from build123d import *

# Parameters (mm, degrees)
ESQUISSE1_W                = 67
ESQUISSE1_H                = 18
BOSS_EXTRU_1_DEPTH         = 3
ESQUISSE2_W                = 10
ESQUISSE2_H                = 3
ENL_V_MAT_EXTRU_1_DEPTH    = 10
R_P_TITION_LIN_AIRE1_COUNT = 4
R_P_TITION_LIN_AIRE1_PITCH = 20
ESQUISSE3_W                = 3
ESQUISSE3_H                = 10
ENL_V_MAT_EXTRU_2_DEPTH    = 10
ESQUISSE4_W                = 3
ESQUISSE4_H                = 10
BOSS_EXTRU_2_DEPTH         = 3


with BuildPart() as part:
    # Esquisse1 → Boss.-Extru.1 (new body)
    with BuildSketch(Plane.XY):
        with Locations((33.5, -9)):
            Rectangle(ESQUISSE1_W, ESQUISSE1_H)
    extrude(amount=BOSS_EXTRU_1_DEPTH)

    # Esquisse2 → Enlèv. mat.-Extru.1 (cut)
    with BuildSketch(Plane.XY.offset(3)):
        with Locations((5, -16.5)):
            Rectangle(ESQUISSE2_W, ESQUISSE2_H)
    enl_v_mat_extru_1 = extrude(amount=-ENL_V_MAT_EXTRU_1_DEPTH, mode=Mode.SUBTRACT)

    # Répétition linéaire1: Enlèv. mat.-Extru.1 ×4
    with Locations(*[(i * R_P_TITION_LIN_AIRE1_PITCH, 0, 0) for i in range(1, R_P_TITION_LIN_AIRE1_COUNT)]):
        add(enl_v_mat_extru_1, mode=Mode.SUBTRACT)

    # Esquisse3 → Enlèv. mat.-Extru.2 (cut)
    with BuildSketch(Plane.XY.offset(3)):
        with Locations((65.5, -5)):
            Rectangle(ESQUISSE3_W, ESQUISSE3_H)
    extrude(amount=-ENL_V_MAT_EXTRU_2_DEPTH, mode=Mode.SUBTRACT)

    # Esquisse4 → Boss.-Extru.2 (add)
    with BuildSketch(Plane.ZY):
        with Locations((1.5, -5)):
            Rectangle(ESQUISSE4_W, ESQUISSE4_H)
    extrude(amount=BOSS_EXTRU_2_DEPTH)


solid = part.part
The listing builds one solid part. Answer for the finished solid, in the listing's coordinates (mm). A direction names the side the tool comes from. Give positions to 0.01 mm unless a question says otherwise; leave off trailing zeros. Write each loop counter-clockwise with the first axis right and the second up, starting at its lowest first coordinate (ties: lowest second). Pieces come first, ordered by that corner, then holes. Notation, with made-up numbers: (62, -40) -> (97, -40) arc R31 ccw to (97, -4) -> close; hole circle Ø1 at (56.5, 33.5). An arc over 180 degrees is marked (long way). Use a Markdown table: item, result.
(1) For faces 4 (the flat face through (63, -15, 2)), 5 (the flat face through (50, -17, 2)), 6 (the flat face through (0, -13, 1)), 7 (the flat face through (64, -5, 2)), determine the directions among +Z, -Z, +X, -X, +Y, -Y from which every point of the face is accessible in a straight line to the end or side of a thin tool.
Return value:
| item | result |
|---|---|
| face 4 | +Z, -Z, +X, -Y |
| face 5 | +Z, -Z, -Y |
| face 6 | +Z, -Z, -X, -Y |
| face 7 | +Z, -Z, +X, +Y |
(2) Determine the mould class of faces 1 (the flat face through (60, -17, 2)), 2 (the flat face through (30, -17, 2)), 3 (the flat face through (65, -10, 2)) for opening direction X: released by +X, released by -X, zero draft, split by the parting line, or undercut.
Return value:
| item | result |
|---|---|
| face 1 | released by +X |
| face 2 | undercut |
| face 3 | zero draft |
(3) Section B-B, the plane y = -3.25 is taken. Determine the outline of the cut face in (x, z), then the cut area to 3 significant figures.
Return value:
| item | result |
|---|---|
| outline | (-3, 0) -> (64, 0) -> (64, 3) -> (-3, 3) -> close |
| area | 201 mm2 |
(4) Section C-C, the plane x = 25.5 is taken. Determine the outline of the cut face in (y, z), then the cut area to 3 significant figures.
Return value:
| item | result |
|---|---|
| outline | (-15, 0) -> (0, 0) -> (0, 3) -> (-15, 3) -> close |
| area | 45.0 mm2 |
(5) Find the intervals of material crossed by probe 1 along X at (y, z) = (-17, 1.4); probe 2 along Y at (x, z) = (2.5, 0.7); probe 3 along X at (y, z) = (-9.5, 1.5), in increasing order. Write a range as from..to.
Return value:
| item | result |
|---|---|
| probe 1 | 10..20, 30..40, 50..60 |
| probe 2 | -15..0 |
| probe 3 | -3..64 |
(6) Flat-ended cylindrical pins translate along their axes: P1, Ø1.5, axis at y = -16, z = 1, coming from the -X side; P2, Ø1.5, axis at y = -11.5, z = 1.5, coming from the -X side; P3, Ø1.5, axis at x = -1.5, z = 1.5, coming from the -Y side. Find the tip coordinate at first contact, or state that the pin passes through.
Return value:
| item | result |
|---|---|
| P1 | x = 10 |
| P2 | x = 0 |
| P3 | y = -10 |
(7) Section A-A, the plane z = 1 is taken. Determine the outline of the cut face in (x, y), then the cut area to 4 significant figures.
Return value:
| item | result |
|---|---|
| outline | (-3, -10) -> (0, -10) -> (0, -15) -> (10, -15) -> (10, -18) -> (20, -18) -> (20, -15) -> (30, -15) -> (30, -18) -> (40, -18) -> (40, -15) -> (50, -15) -> (50, -18) -> (60, -18) -> (60, -15) -> (67, -15) -> (67, -10) -> (64, -10) -> (64, 0) -> (-3, 0) -> close |
| area | 1,095 mm2 |
